from build123d import *

# Parameters (mm, degrees)
CROQUIS2_R               = 2.5
SALIENTE_EXTRUIR1_DEPTH  = 8
BOSS_EXTRUDE1_DEPTH      = 8
CUT_EXTRUDE1_DEPTH       = 8
CUT_EXTRUDE2_DEPTH       = 8
CUT_EXTRUDE3_DEPTH       = 8
BOSS_EXTRUDE2_DEPTH      = 19
BOSS_EXTRUDE2_DEPTH_BACK = 28


with BuildPart() as part:
    # Croquis2 → Saliente-Extruir1 (new body)
    with BuildSketch(Plane(origin=(0, 0, 0), x_dir=(1, 0, 0), z_dir=(0, 1, 0))):
        with BuildLine():
            Line((10.408146681, 33.484891271), (-2.565348209, 122.544918389))
            Line((-2.565348209, 122.544918389), (-6.5, 114.275467894))
            Line((-6.5, 114.275467894), (-6.5, 70))
            Line((-6.5, 70), (-6.5, 0))
            ThreePointArc((-6.5, 0), (0, -6.5), (6.5, 0))
            Line((6.5, 0), (6.5, 24))
            ThreePointArc((6.5, 24), (7.515319953, 29.129248797), (10.408146681, 33.484891271))
        make_face()
        with Locations(Location((0, 0, 0), (0, 0, 270))):
            Circle(CROQUIS2_R, mode=Mode.SUBTRACT)
        with Locations(Location((0, 30, 0), (0, 0, 270))):
            Circle(CROQUIS2_R, mode=Mode.SUBTRACT)
    extrude(amount=SALIENTE_EXTRUIR1_DEPTH)

    # Sketch1 → Boss-Extrude1 (add)
    with BuildSketch(Plane(origin=(0, 0, 0), x_dir=(-1, 0, 0), z_dir=(0, -1, 0))):
        with BuildLine():
            ThreePointArc((4.128942059, -5.020143173), (21.647746033, 11.328640903), (24.761644954, 35.087741621))
            Line((24.761644954, 35.087741621), (6.5, 114.275467894))
            Line((6.5, 114.275467894), (6.5, 0))
            ThreePointArc((6.5, 0), (6.46955751, -0.628351518), (6.378515191, -1.250817318))
            ThreePointArc((6.378515191, -1.250817318), (5.581542691, -3.331123112), (4.128942059, -5.020143173))
        make_face()
    extrude(amount=-BOSS_EXTRUDE1_DEPTH)

    # Sketch2 → Cut-Extrude1 (cut)
    with BuildSketch(Plane(origin=(0, 0, 0), x_dir=(-1, 0, 0), z_dir=(0, -1, 0))):
        with BuildLine():
            Line((17.370234703, 17.816064827), (20.022873599, 19.251371951))
            ThreePointArc((20.022873599, 19.251371951), (13.643712801, 37.157358361), (-3.528479472, 45.308054917))
            Line((-3.528479472, 45.308054917), (-3.528479472, 41.585393249))
            ThreePointArc((-3.528479472, 41.585393249), (11.843666716, 34.028994462), (17.370234703, 17.816064827))
        make_face()
    extrude(amount=-CUT_EXTRUDE1_DEPTH, mode=Mode.SUBTRACT)

    # Sketch3 → Cut-Extrude2 (cut)
    with BuildSketch(Plane(origin=(0, 0, 0), x_dir=(-1, 0, 0), z_dir=(0, -1, 0))):
        with BuildLine():
            Line((13.617187508, 49.133891817), (16.20693955, 49.133891817))
            ThreePointArc((16.20693955, 49.133891817), (8.831529271, 57.239594637), (-2.115270782, 57.755989445))
            Line((-2.115270782, 57.755989445), (-2.115270782, 56.050896345))
            ThreePointArc((-2.115270782, 56.050896345), (7.183516906, 55.850692877), (13.617187508, 49.133891817))
        make_face()
    extrude(amount=-CUT_EXTRUDE2_DEPTH, mode=Mode.SUBTRACT)

    # Sketch4 → Cut-Extrude3 (cut)
    with BuildSketch(Plane(origin=(0, 0, 0), x_dir=(-1, 0, 0), z_dir=(0, -1, 0))):
        with BuildLine():
            Line((11.367603777, 69.893539148), (13.075452067, 70.772160082))
            ThreePointArc((13.075452067, 70.772160082), (8.326822135, 77.799434944), (0, 79.410680226))
            Line((0, 79.410680226), (0, 76.04148357))
            ThreePointArc((0, 76.04148357), (6.957082869, 75.321819187), (11.367603777, 69.893539148))
        make_face()
    extrude(amount=-CUT_EXTRUDE3_DEPTH, mode=Mode.SUBTRACT)

    # Sketch5 → Boss-Extrude2 (add, two sides: drawn at the far end of the back side and taken through both)
    with BuildSketch(Plane(origin=(0, 0, 0), x_dir=(-1, 0, 0), z_dir=(0, -1, 0)).offset(-BOSS_EXTRUDE2_DEPTH_BACK)):
        Polygon((-9.233196645, 41.550650182), (1.963037177, 118.410193142), (4.819417727, 117.807544593), (-4.03262502, 41.550650182), align=None)
    extrude(amount=BOSS_EXTRUDE2_DEPTH + BOSS_EXTRUDE2_DEPTH_BACK)


solid = part.part
Part model, mm, in its own coordinate system. A direction names the side the tool comes from. Coordinates: 2 decimals unless noted, no trailing zeros. Loops run counter-clockwise (first coordinate to the right, second up) from the corner with the lowest first, then second, coordinate; pieces in that order, holes last. Notation, with made-up numbers: (22.5, 56) -> (61.5, 56) arc R10 ccw to (61.5, 72) -> close; hole circle Ø6 at (83.5, 20). An arc over 180 degrees is marked (long way). Use a Markdown table: item, result. Add a question column.
Item 1: Band-saw the part on D-D on y = 15. Write the cut outline in (x, z), plus the area to 3 significant figures.
Item 2: Band-saw the part on B-B on x = -8. Write the cut outline in (y, z), plus the area to 3 significant figures.
Item 3: Flat gauge pins, fed straight in: P1, Ø8, axis at x = -22, z = -57, coming from the -Y side; P2, Ø8, axis at x = 0.5, y = 18.5, coming from the -Z side; P3, Ø2.5, axis at y = 4.5, z = -9.5, coming from the +X side. Where does each tip first touch, or does it go through?
Item 4: Band-saw the part on C-C on z = -30. Write the cut outline in (x, y), plus the area to 3 significant figures.
Item 5: Probe probe 1 along X at (y, z) = (7, -31.5); probe 2 along Y at (x, z) = (-16, -71.5); probe 3 along X at (y, z) = (4, -30). List the from-to ranges inside material, lowest first.
Item 6: Band-saw the part on A-A on z = -53.5. Write the cut outline in (x, y).
Item 7: Which spindle directions (+Z, -Z, +X, -X, +Y, -Y) get a long thin tool onto all of the face, cutting with end or side? Do faces 4 (the flat face through (-7, 0, -43)), 5 (the flat face through (7, 18, -41.551)), 6 (the flat face through (-7, 8, -43)), 7 (the cylindrical face through (-13.83, 3.94, -36.95)). Say none if no direction does.
Item 8: Pull direction X, two halves, no side cores. Call faces 1 (the flat face through (6.5, 4, -12)), 2 (the flat face through (-3, 8, -120)), 3 (the cylindrical face through (-7.061, 3.944, -55.904)): +X half, -X half, draft (parallel to the pull), parting line (faces both ways), or undercut.
Geometry says:
| question | item | result |
|---|---|---|
| 1 | outline | (-4.82, -117.81) -> (-1.96, -118.41) -> (9.23, -41.55) -> (4.03, -41.55) -> close |
| 1 | area | 311 mm² |
| 2 | outline | (0, -107.77) -> (8, -107.77) -> (8, -78.01) -> (0, -78.01) -> close; (0, -74.66) -> (8, -74.66) -> (8, -57.6) -> (0, -57.6) -> close; (0, -55.45) -> (8, -55.45) -> (8, -41.8) -> (0, -41.8) -> close; (0, -37.49) -> (8, -37.49) -> (8, 3.07) -> (0, 3.07) -> close |
| 2 | area | 808 mm² |
| 3 | P1 | y = 0 |
| 3 | P2 | z = -118.41 |
| 3 | P3 | x = 6.5 |
| 4 | outline | (-25.49, 0) -> (-18.17, 0) -> (-18.17, 8) -> (-25.49, 8) -> close; (-14.67, 0) -> (-2.5, 0) -> (-2.5, 8) -> (-14.67, 8) -> close; (2.5, 0) -> (7.91, 0) -> (7.91, 8) -> (2.5, 8) -> close |
| 4 | area | 199 mm² |
| 5 | probe 1 | -25.35 to -17.49, -13.77 to -2, 2 to 8.78 |
| 5 | probe 2 | 0 to 8 |
| 5 | probe 3 | -25.49 to -18.17, -14.67 to -2.5, 2.5 to 7.91 |
| 6 | outline | (-20.52, 0) -> (-13.69, 0) -> (-13.69, 8) -> (-20.52, 8) -> close; (-10.7, 0) -> (2.65, 0) -> (2.65, -19) -> (7.49, -19) -> (7.49, 28) -> (2.65, 28) -> (2.65, 8) -> (-10.7, 8) -> close |
| 7 | face 4 | +Z, -X, -Y |
| 7 | face 5 | +Z, +X, -X, +Y |
| 7 | face 6 | +Z, -X, +Y |
| 7 | face 7 | +Y, -Y |
| 8 | face 1 | +X half |
| 8 | face 2 | draft |
| 8 | face 3 | undercut |
